Could you check a few things on this model? Use its own coordinates, in mm. A direction names the side the tool comes from. Coordinates: 2 decimals unless noted, no trailing zeros. Order: outer loops, then holes, each group sorted by start corner. A loop starts at its lowest first (then second) coordinate and runs counter-clockwise, first axis right, second up. Notation, with made-up numbers: (55.25, 36) -> (75.25, 36) arc R22 ccw to (75.25, 54) -> close; hole circle Ø2 at (44, 75). An arc over 180 degrees is marked (long way). Use a Markdown table: item, result. Add a question column.
1) If we section it at A-A (z = -132.5): Write out the boundary of the cut face in (x, y) (3 decimals), plus the area to 3 significant figures.
2) If I drill on L1, parallel to Y at x = 137, z = -240 (3 decimals); L2, parallel to Z at x = 144.5, y = -14; L3, parallel to Z at x = 170, y = -1.5, over which ranges is the centre line in solid material (lowest first)? Write a range as [from, to].
3) Which directions (+Z, -Z, +X, -X, +Y, -Y) give clear straight access to the entire face, cutting with the end or side of a thin tool? Please do faces 4 (the flat face through (148, -22, -294.132)), 5 (the cylindrical face through (98.499, -1.565, -225.825)).
4) Will these pins go through, and if not, where does the flat tip stop? pin 1 Ø1.6 at (x, y) = (328.5, -1) entering from -Z; pin 2 Ø3 at (x, y) = (230.5, -14) entering from +Z; pin 3 Ø5 at (x, z) = (170.5, -133) entering from -Y (3 decimals); pin 4 Ø3 at (x, z) = (177.5, -131) entering from +Y.
5) Thinking about a two-plate mould opening in X: for faces 1 (the cylindrical face through (126.95, -1.57, -103.02)), 2 (the flat face through (102.02, -1.57, -36.35)), 3 (the flat face through (148, -22, -297.307)), which applies, +X half, -X half, draft (parallel to the pull), parting line (faces both ways), or undercut?
6) If we section it at B-B (x = 328.5): Write out the boundary of the cut face in (y, z) (3 decimals), plus the area to 3 significant figures.
```python
from build123d import *

# Parameters (mm, degrees)
BASE_FLANGE1_DEPTH = 3.175
EDGE_FLANGE1_DEPTH = 197.512880056
SKETCH9_R          = 12.065
CUT_EXTRUDE1_DEPTH = 3.175


# Sheet-metal steps are written as plain solids
with BuildPart() as part:
    # Sketch1 → Base-Flange1 (new body)
    with BuildSketch(Plane(origin=(0, 0, 0), x_dir=(1, 0, 0), z_dir=(0, 1, 0))):
        Polygon((154.686, -16.51), (355.6, -16.51), (355.6, 290.957), (50.8, 290.957), (50.8, 87.757), align=None)
    extrude(amount=-BASE_FLANGE1_DEPTH)

    # Edge-Flange1 section (across the edge) → Edge-Flange1 (add)
    with BuildSketch(Plane(origin=(50.8, -3.175, -294.132), x_dir=(0, 0, 1), z_dir=(1, 0, 0))):
        with BuildLine():
            Line((-3.175, 3.175), (-3.175, 34.925))
            Line((-3.175, 34.925), (0, 34.925))
            Line((0, 34.925), (0, 3.175))
            ThreePointArc((0, 3.175), (0.92993597, 0.92993597), (3.175, 0))
            Line((3.175, 0), (3.175, -3.175))
            ThreePointArc((3.175, -3.175), (-1.315128061, -1.315128061), (-3.175, 3.175))
        make_face()
    extrude(amount=EDGE_FLANGE1_DEPTH)

    # Sketch9 → Cut-Extrude1 (cut)
    with BuildSketch(Plane(origin=(0, 0, 0), x_dir=(1, 0, 0), z_dir=(0, 1, 0))):
        with BuildLine():
            ThreePointArc((84.925, 225.833155379), (83.375, 227.383155379), (81.825, 225.833155379))
            ThreePointArc((81.825, 225.833155379), (83.375, 224.283155379), (84.925, 225.833155379))
        make_face()
        with BuildLine():
            ThreePointArc((104.825, 225.833155379), (106.375, 224.283155379), (107.925, 225.833155379))
            ThreePointArc((107.925, 225.833155379), (106.375, 227.383155379), (104.825, 225.833155379))
        make_face()
        with BuildLine():
            ThreePointArc((104.825, 248.833155379), (106.375, 247.283155379), (107.925, 248.833155379))
            ThreePointArc((107.925, 248.833155379), (106.375, 250.383155379), (104.825, 248.833155379))
        make_face()
        with BuildLine():
            ThreePointArc((84.925, 248.833155379), (83.375, 250.383155379), (81.825, 248.833155379))
            ThreePointArc((81.825, 248.833155379), (83.375, 247.283155379), (84.925, 248.833155379))
        make_face()
        with Locations(Location((94.875, 237.333155379, 0), (0, 0, 270))):
            Circle(SKETCH9_R)
        with BuildLine():
            ThreePointArc((136.36996, 79.466155379), (137.91996, 77.916155379), (139.46996, 79.466155379))
            ThreePointArc((139.46996, 79.466155379), (137.91996, 81.016155379), (136.36996, 79.466155379))
        make_face()
        with BuildLine():
            ThreePointArc((136.36996, 102.466155379), (137.91996, 100.916155379), (139.46996, 102.466155379))
            ThreePointArc((139.46996, 102.466155379), (137.91996, 104.016155379), (136.36996, 102.466155379))
        make_face()
        with Locations(Location((126.41996, 90.966155379, 0), (0, 0, 270))):
            Circle(SKETCH9_R)
        with BuildLine():
            ThreePointArc((113.36996, 102.466155379), (114.91996, 100.916155379), (116.46996, 102.466155379))
            ThreePointArc((116.46996, 102.466155379), (114.91996, 104.016155379), (113.36996, 102.466155379))
        make_face()
        with BuildLine():
            ThreePointArc((113.36996, 79.466155379), (114.91996, 77.916155379), (116.46996, 79.466155379))
            ThreePointArc((116.46996, 79.466155379), (114.91996, 81.016155379), (113.36996, 79.466155379))
        make_face()
    extrude(amount=-CUT_EXTRUDE1_DEPTH, mode=Mode.SUBTRACT)


solid = part.part
```
Answer sheet:
| question | item | result |
|---|---|---|
| 1 | outline | (50.8, -3.175) -> (355.6, -3.175) -> (355.6, 0) -> (50.8, 0) -> close |
| 1 | area | 968 mm2 |
| 2 | L1 | [-3.175, 0] |
| 2 | L2 | [-297.31, -294.13] |
| 2 | L3 | [-295.06, 16.51] |
| 3 | face 4 | +Z, +X, -X, -Y |
| 3 | face 5 | +Y, -Y |
| 4 | pin 1 | z = -290.96 |
| 4 | pin 2 | z = -294.13 |
| 4 | pin 3 | y = -3.175 |
| 4 | pin 4 | y = 0 |
| 5 | face 1 | undercut |
| 5 | face 2 | -X half |
| 5 | face 3 | draft |
| 6 | outline | (-3.175, -290.957) -> (0, -290.957) -> (0, 16.51) -> (-3.175, 16.51) -> close |
| 6 | area | 976 mm2 |
